from build123d import *

# Parameters (mm, degrees)
SKETCH_8_R      = 40
SKETCH_8_R_2    = 1
SKETCH_8_R_3    = 2.6
EXTRUDE_3_DEPTH = 1.6


with BuildPart() as part:
    # 草图8 → 凸台-拉伸3 (new body)
    with BuildSketch(Plane.XY):
        with Locations((-53.736575471, -2.872479928)):
            Circle(SKETCH_8_R)
        with Locations((-53.736575471, 7.500392818)):
            Circle(SKETCH_8_R_2, mode=Mode.SUBTRACT)
        with Locations((-46.735230698, 4.127771963)):
            Circle(SKETCH_8_R_2, mode=Mode.SUBTRACT)
        with Locations((-42.236448471, -2.999480182)):
            Circle(SKETCH_8_R_2, mode=Mode.SUBTRACT)
        with Locations((-46.737760534, -9.869682445)):
            Circle(SKETCH_8_R_2, mode=Mode.SUBTRACT)
        with Locations((-53.736575471, -13.499607182)):
            Circle(SKETCH_8_R_2, mode=Mode.SUBTRACT)
        with Locations((-60.737570724, -9.872335788)):
            Circle(SKETCH_8_R_2, mode=Mode.SUBTRACT)
        with Locations((-65.236448471, -2.999480182)):
            Circle(SKETCH_8_R_2, mode=Mode.SUBTRACT)
        with Locations((-60.73580463, 4.12809202)):
            Circle(SKETCH_8_R_2, mode=Mode.SUBTRACT)
        with Locations((-62.528088914, 29.934409619)):
            Circle(SKETCH_8_R_3, mode=Mode.SUBTRACT)
        with Locations((-44.946804677, 29.93487656)):
            Circle(SKETCH_8_R_3, mode=Mode.SUBTRACT)
        with Locations((-29.720732426, 21.144638825)):
            Circle(SKETCH_8_R_3, mode=Mode.SUBTRACT)
        with Locations((-20.929685924, 5.919033515)):
            Circle(SKETCH_8_R_3, mode=Mode.SUBTRACT)
        with Locations((-20.929218983, -11.662250722)):
            Circle(SKETCH_8_R_3, mode=Mode.SUBTRACT)
        with Locations((-29.719456719, -26.888322973)):
            Circle(SKETCH_8_R_3, mode=Mode.SUBTRACT)
        with Locations((-44.945062029, -35.679369475)):
            Circle(SKETCH_8_R_3, mode=Mode.SUBTRACT)
        with Locations((-62.526346266, -35.679836416)):
            Circle(SKETCH_8_R_3, mode=Mode.SUBTRACT)
        with Locations((-77.752418517, -26.88959868)):
            Circle(SKETCH_8_R_3, mode=Mode.SUBTRACT)
        with Locations((-86.543465018, -11.66399337)):
            Circle(SKETCH_8_R_3, mode=Mode.SUBTRACT)
        with Locations((-86.543931959, 5.917290867)):
            Circle(SKETCH_8_R_3, mode=Mode.SUBTRACT)
        with Locations((-77.753694224, 21.143363118)):
            Circle(SKETCH_8_R_3, mode=Mode.SUBTRACT)
        with BuildLine():
            Line((-58.736575471, 24.6774747), (-58.736575471, 11.269655696))
            ThreePointArc((-58.736575471, 11.269655696), (-66.726956528, 4.627520072), (-68.484024185, -5.613420721))
            Line((-68.484024185, -5.613420721), (-80.095536052, -12.317330223))
            ThreePointArc((-80.095536052, -12.317330223), (-77.985286777, 11.127520072), (-58.736575471, 24.6774747))
        make_face(mode=Mode.SUBTRACT)
        Polygon((-57.085216568, -8.799480182), (-50.277963232, -8.735988313), (-46.929322134, -2.808988059), (-50.387934374, 3.054520326), (-57.195187711, 2.991028458), (-60.543828808, -2.935971796), align=None, mode=Mode.SUBTRACT)
        with BuildLine():
            Line((-48.736575471, 24.6774747), (-48.736575471, 11.269655696))
            ThreePointArc((-48.736575471, 11.269655696), (-40.746194414, 4.627520072), (-38.989126757, -5.613420721))
            Line((-38.989126757, -5.613420721), (-27.37761489, -12.317330223))
            ThreePointArc((-27.37761489, -12.317330223), (-29.487864165, 11.127520072), (-48.736575471, 24.6774747))
        make_face(mode=Mode.SUBTRACT)
        with BuildLine():
            Line((-32.37761489, -20.977584261), (-43.989126757, -14.273674759))
            ThreePointArc((-43.989126757, -14.273674759), (-53.736575471, -17.872479928), (-63.484024185, -14.273674759))
            Line((-63.484024185, -14.273674759), (-75.095536052, -20.977584261))
            ThreePointArc((-75.095536052, -20.977584261), (-53.736575471, -30.872479928), (-32.37761489, -20.977584261))
        make_face(mode=Mode.SUBTRACT)
    extrude(amount=EXTRUDE_3_DEPTH)


solid = part.part
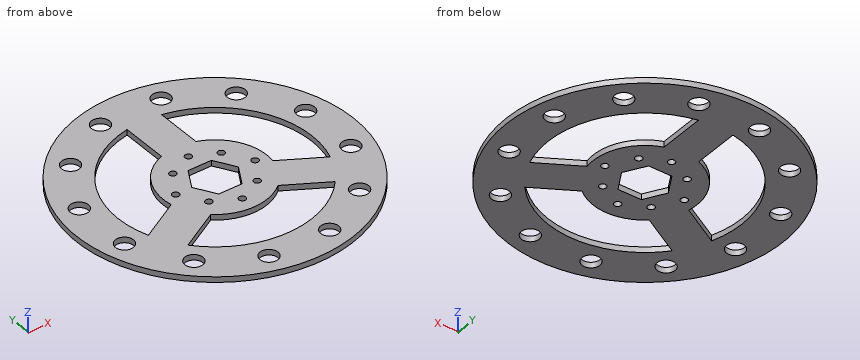
Read the model definition and answer for the solid it produces. Units are mm, in the model's axes. Coordinates: 2 decimals unless noted, no trailing zeros. Loops run counter-clockwise (first coordinate to the right, second up) from the corner with the lowest first, then second, coordinate; pieces in that order, holes last. Notation, with made-up numbers: (78, 52.5) -> (83, 52.5) arc R22 ccw to (83, 83.5) -> close; hole circle Ø5 at (18, 77.25). An arc over 180 degrees is marked (long way). Write item = value, one per line. Start each with the question number.
1) The part is cut by section C-C, the plane z = 0.9. State how many separate pieces and enclosed holes the cut face has, plus the area to 3 significant figures.
2) Find the intervals of material crossed by L1, parallel to Y at x = -67.5, z = 1.4; L2, parallel to X at y = 2, z = 1.45; L3, parallel to X at y = -12, z = 1.2, in increasing order. Write a range as from..to.
3) The part is cut by section A-A, the plane x = -21. Determine the outline of the cut face in (y, z), plus the area to 3 significant figures.
4) The part is cut by section D-D, the plane x = -83. Determine the outline of the cut face in (y, z).
5) The part is cut by section B-B, the plane y = 28.5. Determine the outline of the cut face in (x, z).
Result:
q1.separate_pieces = 1
q1.enclosed_holes = 24
q1.area = 3,260 mm²
q2.L1 = -40.43..-27.26, -16.59..3.09, 21.51..34.69
q2.L2 = -93.44..-81.31, -67.92..-57.76, -49.77..-39.55, -26.16..-14.03
q2.L3 = -92.68..-89.12, -83.97..-80.21, -79.55..-27.93, -27.27..-23.51, -18.35..-14.79
q3.outline = (-25.86, 0) -> (-14.26, 0) -> (-14.26, 1.6) -> (-25.86, 1.6) -> close; (-9.06, 0) -> (3.32, 0) -> (3.32, 1.6) -> (-9.06, 1.6) -> close; (8.52, 0) -> (20.11, 0) -> (20.11, 1.6) -> (8.52, 1.6) -> close
q3.area = 56.9 mm²
q4.outline = (-30.14, 0) -> (24.4, 0) -> (24.4, 1.6) -> (-30.14, 1.6) -> close
q5.outline = (-78.55, 0) -> (-64.7, 0) -> (-64.7, 1.6) -> (-78.55, 1.6) -> close; (-60.36, 0) -> (-47.12, 0) -> (-47.12, 1.6) -> (-60.36, 1.6) -> close; (-42.78, 0) -> (-28.92, 0) -> (-28.92, 1.6) -> (-42.78, 1.6) -> close
